Source: CAD feature listing. Evaluate the final solid. Frame: model axes, mm. A direction names the side the tool comes from. Give positions to 0.01 mm unless a question says otherwise; leave off trailing zeros. Order: outer loops, then holes, each group sorted by start corner. A loop starts at its lowest first (then second) coordinate and runs counter-clockwise, first axis right, second up. Notation, with made-up numbers: M 66.25,47 L 102.25,47 A14 ccw 102.25,51 Z; hole C 65.25,36.5 d7. An arc over 180 degrees is marked long. Answer as a JSON object with one key per item and string values. Group by question number.
1. Set-up query: faces 1 (the cylindrical face through (19, -20, 11)), 2 (the cylindrical face through (17.5, -4.5, 6.1)), 3 (the cylindrical face through (-2.4, -16.1, 14.2)). Return all of +Z, -Z, +X, -X, +Y, -Y with unobstructed straight access to the full face (end or side cutting, diameter ignored); none if empty.
2. Section query D-D (z = 6). Output: boundary loops of the cut face in (x, y), plus the area to 3 significant figures.
3. Pin query (flat end, axial travel): P1, Ø4, axis at x = 0.5, z = 11, coming from the -Y side. Return the tip coordinate at first contact, or that it passes through.
4. Pull-direction query (Y, two-part tool) for faces 4 (the cylindrical face through (19, 20, 11)), 5 (the flat face through (0, 0, 0)), 6 (the flat face through (14, 0, 6)); classes: +Y half, -Y half, draft (parallel to the pull), parting line (faces both ways), or undercut.
5. Section query B-B (y = 1). Output: boundary loops of the cut face in (x, z).
6. Material intervals for L1, parallel to X at y = -15.5, z = 11; L2, parallel to Y at x = 16.5, z = 5.5; L3, parallel to Y at x = 2, z = 14, sorted ascending. Write a range as [from, to].
7. Section query C-C (x = 0). Output: boundary loops of the cut face in (y, z), plus the area to 3 significant figures.
8. Section query A-A (z = 11). Output: boundary loops of the cut face in (x, y), plus the area to 3 significant figures.
from build123d import *

# Parameters (mm, degrees)
SKETCH_1_W          = 42
SKETCH_1_H          = 42
EXTRUDE_1_DEPTH     = 22
SKETCH_2_R          = 1.5
CUT_EXTRUDE_1_DEPTH = 7
SKETCH_3_R          = 4
CUT_EXTRUDE_2_DEPTH = 10
FILLET_1_R          = 5


with BuildPart() as part:
    # 草图1 → 凸台-拉伸1 (new body)
    with BuildSketch(Plane.XY):
        Rectangle(SKETCH_1_W, SKETCH_1_H)
    extrude(amount=EXTRUDE_1_DEPTH)

    # 草图2 → 切除-拉伸1 (cut)
    with BuildSketch(Plane(origin=(21, 0, 0), x_dir=(0, 0, -1), z_dir=(1, 0, 0))):
        with Locations((-6.07507845, 3)):
            Circle(SKETCH_2_R)
        with BuildLine():
            ThreePointArc((-4.57507845, 3), (-6.07507845, 1.5), (-7.57507845, 3))
            Line((-7.57507845, 3), (-7.57507845, -3))
            ThreePointArc((-7.57507845, -3), (-6.07507845, -1.5), (-4.57507845, -3))
            Line((-4.57507845, -3), (-4.57507845, 3))
        make_face()
        with Locations((-6.07507845, -3)):
            Circle(SKETCH_2_R)
    extrude(amount=-CUT_EXTRUDE_1_DEPTH, mode=Mode.SUBTRACT)

    # 草图3 → 切除-拉伸2 (cut)
    with BuildSketch(Plane.XZ.offset(21)):
        with Locations(Location((0, 11, 0), (0, 0, 270))):
            Circle(SKETCH_3_R)
    extrude(amount=-CUT_EXTRUDE_2_DEPTH, mode=Mode.SUBTRACT)

    # 圆角1
    fillet_1_edges = [part.edges().sort_by_distance(p)[0] for p in [
        (-21, 21, 11),
        (21, 21, 11),
        (21, -21, 11),
        (-21, -21, 11),
    ]]
    fillet(fillet_1_edges, radius=FILLET_1_R)


solid = part.part
Answer sheet:
{
 "1": {"face 1": "+Z, -Z, +X, -Y", "face 2": "+X", "face 3": "-Y"},
 "2": {"outline": "M -21,-16 A5 ccw -16,-21 L 16,-21 A5 ccw 21,-16 L 21,-4.5 L 14,-4.5 L 14,4.5 L 21,4.5 L 21,16 A5 ccw 16,21 L -16,21 A5 ccw -21,16 Z", "area": "1,680 mm^2"},
 "3": {"P1": "y = -11"},
 "4": {"face 4": "+Y half", "face 5": "draft", "face 6": "undercut"},
 "5": {"outline": "M -21,0 L 21,0 L 21,4.58 L 14,4.58 L 14,7.58 L 21,7.58 L 21,22 L -21,22 Z"},
 "6": {"L1": "[-21, -4], [4, 21]", "L2": "[-20.97, -4.39], [4.39, 20.97]", "L3": "[-11, 21]"},
 "7": {"outline": "M -21,0 L 21,0 L 21,22 L -21,22 L -21,15 L -11,15 L -11,7 L -21,7 Z", "area": "844 mm^2"},
 "8": {"outline": "M -21,-16 A5 ccw -16,-21 L -4,-21 L -4,-11 L 4,-11 L 4,-21 L 16,-21 A5 ccw 21,-16 L 21,16 A5 ccw 16,21 L -16,21 A5 ccw -21,16 Z", "area": "1,660 mm^2"}
}
